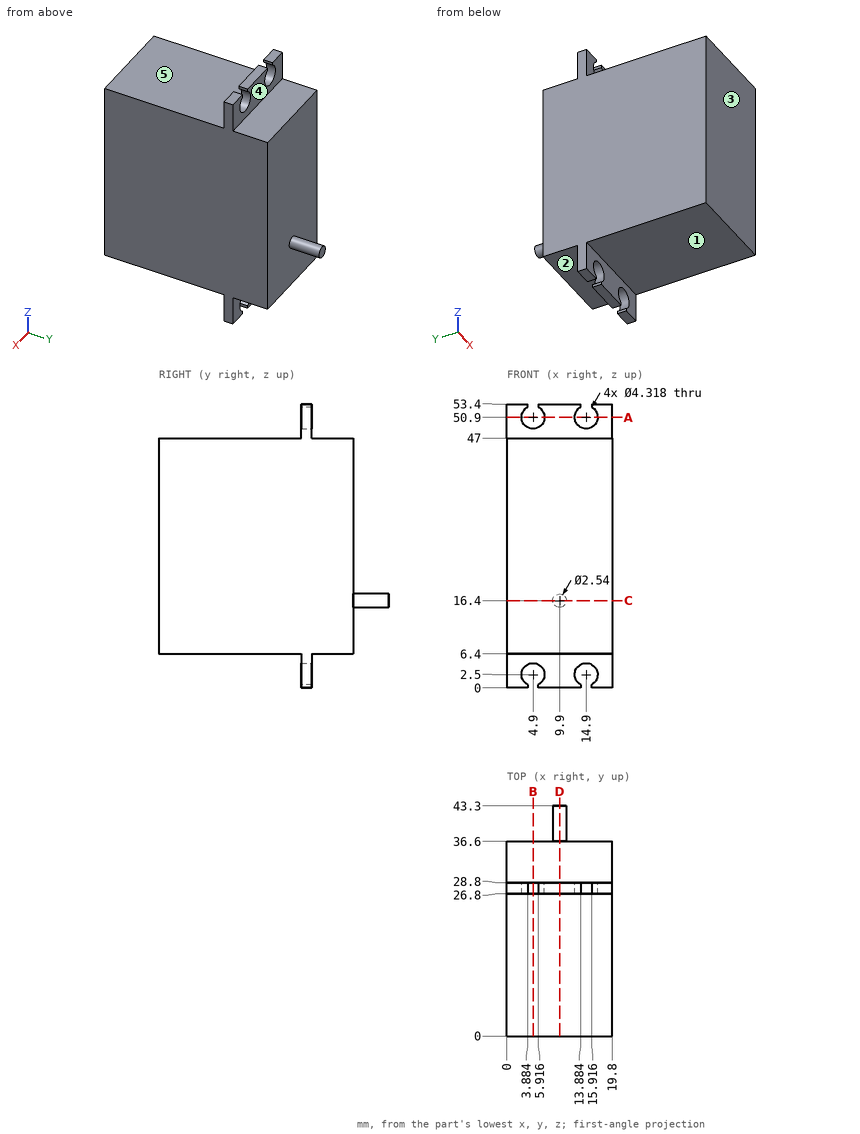
Job drawing, mm, ordinate dimensions from the low corner. One solid piece. A direction names the side the tool comes from. Round coordinates to 2 decimals unless told otherwise and drop trailing zeros. Loops run counter-clockwise (first coordinate to the right, second up) from the corner with the lowest first, then second, coordinate; pieces in that order, holes last. Notation, with made-up numbers: (-34.5, -14) -> (-0.5, -14) arc R22 cw to (-0.5, 19) -> close; hole circle Ø11 at (-10, 82.5). An arc over 180 degrees is marked (long way). Use CSV: the item, a comma, the result in double quotes. Start each with the question number.
Q1. Saw through at D-D on x = 9.9. Give the cut face in (y, z), and give its area (3 significant figures).
Q2. Flat gauge pins, fed straight in: pin 1 Ø5.5 at (x, z) = (4.9, 50.9) entering from -Y; pin 2 Ø3 at (x, y) = (14.5, 12.5) entering from -Z; pin 3 Ø2.5 at (x, z) = (14.9, 50.9) entering from +Y; pin 4 Ø10 at (x, y) = (11, 16) entering from +Z. Where does each tip first touch, or does it go through?
Q3. Which spindle directions (+Z, -Z, +X, -X, +Y, -Y) get a long thin tool onto all of the face, cutting with end or side? Do the marked faces 1, 2, 3, 4 and 5. Say none if no direction does.
Q4. Saw through at C-C on z = 16.4. Give the cut face in (x, y).
Q5. Drill centre lines: L1, parallel to X at y = 27.8, z = 50.9; L2, parallel to X at y = 27, z = 50; L3, parallel to Z at x = 4.9, y = 27.65. Where is each one in solid material? Low to high.
Q6. Saw through at B-B on x = 4.9. Give the cut face in (y, z).
Q7. Saw through at A-A on z = 50.9. Give the cut face in (x, y), and give its area (3 significant figures).
Solutions:
1,outline,"(0, 6.4) -> (26.8, 6.4) -> (26.8, 0) -> (28.8, 0) -> (28.8, 6.4) -> (36.6, 6.4) -> (36.6, 15.13) -> (43.3, 15.13) -> (43.3, 17.67) -> (36.6, 17.67) -> (36.6, 47) -> (28.8, 47) -> (28.8, 53.4) -> (26.8, 53.4) -> (26.8, 47) -> (0, 47) -> close"
1,area,"1,530 mm^2"
2,pin 1,"stops at y = 26.8"
2,pin 2,"stops at z = 6.4"
2,pin 3,"passes through"
2,pin 4,"stops at z = 47"
3,face 1,"-Z, +X, -X, -Y"
3,face 2,"-Z, +X, -X, +Y"
3,face 3,"+Z, -Z, +X, -X, -Y"
3,face 4,"+Z, +X, -X, +Y"
3,face 5,"+Z, +X, -X, -Y"
4,outline,"(0, 0) -> (19.8, 0) -> (19.8, 36.6) -> (11.17, 36.6) -> (11.17, 43.3) -> (8.63, 43.3) -> (8.63, 36.6) -> (0, 36.6) -> close"
5,L1,"x = 0 to 2.74, 7.06 to 12.74, 17.06 to 19.8"
5,L2,"x = 0 to 2.94, 6.86 to 12.94, 16.86 to 19.8"
5,L3,"z = 4.66 to 48.74"
6,outline,"(0, 6.4) -> (26.8, 6.4) -> (26.8, 4.66) -> (28.8, 4.66) -> (28.8, 6.4) -> (36.6, 6.4) -> (36.6, 47) -> (28.8, 47) -> (28.8, 48.74) -> (26.8, 48.74) -> (26.8, 47) -> (0, 47) -> close"
7,outline,"(0, 26.8) -> (2.74, 26.8) -> (2.74, 28.8) -> (0, 28.8) -> close; (7.06, 26.8) -> (12.74, 26.8) -> (12.74, 28.8) -> (7.06, 28.8) -> close; (17.06, 26.8) -> (19.8, 26.8) -> (19.8, 28.8) -> (17.06, 28.8) -> close"
7,area,"22.3 mm^2"
